For this review, take the finished solid that the model builds, in its own axes (mm). A direction names the side the tool comes from. Give positions to 0.01 mm unless a question says otherwise; leave off trailing zeros. Loops run counter-clockwise (first coordinate to the right, second up) from the corner with the lowest first, then second, coordinate; pieces in that order, holes last. Notation, with made-up numbers: (-17, 32.5) - (38, 32.5) arc R20 cw to (38, 49.5) - close; hole circle Ø4 at (-18.75, 78). An arc over 180 degrees is marked (long way). Answer as CSV lines item,"result".
Autodesk Inventor part; units mm, degrees
ref_plane "YZ Plane" through (0, 0, 0) normal (1, 0, 0) x (0, 1, 0)
ref_plane "XZ Plane" through (0, 0, 0) normal (0, 1, 0) x (-1, 0, 0)
ref_plane "XY Plane" through (0, 0, 0) normal (0, 0, 1) x (1, 0, 0)
sketch "Sketch1" plane through (0, 0, 0) normal (0, 0, 1) x (1, 0, 0)
  line L0 (0, 0) -> (18, 0)
  line L1 (18, 0) -> (18, 13)
  line L2 (18, 13) -> (12, 13)
  line L3 (12, 13) -> (12, 3)
  line L4 (12, 3) -> (0, 3)
  line L5 (0, 3) -> (0, 0) construction
  line L6 (0, 0) -> (-18, 0)
  line L7 (-18, 0) -> (-18, 13)
  line L8 (-18, 13) -> (-12, 13)
  line L9 (-12, 13) -> (-12, 3)
  line L10 (-12, 3) -> (0, 3)
  point P0 (15, 13)
  dimension "d2" = 6
  dimension "d3" = 3
  dimension "d4" = 13
  dimension "d18" = 15
extrude "Extrusion1" add sketch "Sketch1" along normal blind 12
sketch "Sketch2" plane through (-18, 0, 0) normal (0, -1, 0) x (1, 0, 0)
  circle A0 centre (18, 6) radius 1.1
  line L0 (0, 0) -> (36, 0)
  line L1 (0, 0) -> (0, 12)
  point P0 (18, 0)
  dimension "d7" = 2.2
  dimension "d19" = 6
  dimension "d20" = 18
extrude "Extrusion2" cut sketch "Sketch2" against normal blind 12
sketch "Sketch3" plane through (-12, 3, 0) normal (0, 1, 0) x (1, 0, 0)
  circle A0 centre (12, -6) radius 1.1
  circle A1 centre (12, -6) radius 4
  point P0 (12, 0)
  dimension "d11" = 8
extrude "Extrusion3" add sketch "Sketch3" along normal blind 7
sketch "Sketch5" plane through (0, 0, 0) normal (0, 0, -1) x (-1, 0, 0)
  circle A0 centre (0, 6.6873) radius 1.1
  line L0 (-12, 3) -> (12, 3)
  point P0 (0, 3)
  dimension "d29" = 2.2
extrude "Extrusion5" cut sketch "Sketch5" against normal blind 5.75
equation "\"d19\" = 0.5 * d5"
equation "\"d20\" = d18 + 0.5 * d2"
properties part number "Support_Holder" material "ABS Plastic"
1) Machinability: for faces 4 (the cylindrical face through (-1.05, 7.02, 3.43)), 5 (the cylindrical face through (2.15, 6.451, 9.373)), 6 (the flat face through (12, 8, 6)), 7 (the flat face through (15, 13, 6)), 8 (the flat face through (18, 6, 6)), which of the approach directions +Z, -Z, +X, -X, +Y, -Y give a long, thin tool a straight path to every point of the face, cutting with its end or side? Answer none if there is none.
From the geometry:
face 4,"-Z"
face 5,"+Y"
face 6,"+Z, -Z, +Y"
face 7,"+Z, -Z, +X, -X, +Y"
face 8,"+Z, -Z, +X, +Y, -Y"
2) Consider section A-A on y = 3.5. Write out the cut boundary in (x, z).
From the geometry:
outline,"(-18, 0) - (-12, 0) - (-12, 12) - (-18, 12) - close; circle Ø8 at (0, 6); (12, 0) - (18, 0) - (18, 12) - (12, 12) - close; hole circle Ø2.2 at (0, 6)"
3) Wall thickness on line 1 (X direction, y = 7, z = 6); line 2 (X direction, y = 12, z = 0.75); line 3 (X direction, y = 9.5, z = 3.75): over which ranges is each line inside the solid? List them lowest first. Write a range as from..to.
From the geometry:
line 1,"x = -18..-12, -4..-1.1, 1.1..4, 12..18"
line 2,"x = -18..-12, 12..18"
line 3,"x = -18..-12, -3.31..3.31, 12..18"
4) Draft analysis for pull direction X (two halves, no side actions). For faces 1 (the flat face through (-4, 2, 12)), 2 (the flat face through (-18, 6, 6)), 3 (the flat face through (-12, 8, 6)), state which applies: pulls with the +X half, pulls with the -X half, needs draft (parallel to the pull), parting line crosses it, or undercut.
From the geometry:
face 1,"needs draft"
face 2,"pulls with the -X half"
face 3,"undercut"
5) Consider section D-D on z = 7.5. Write out the cut boundary in (x, y), and give its area (3 significant figures).
From the geometry:
outline,"(-18, 0) - (18, 0) - (18, 13) - (12, 13) - (12, 3) - (3.71, 3) - (3.71, 10) - (-3.71, 10) - (-3.71, 3) - (-12, 3) - (-12, 13) - (-18, 13) - close"
area,"280 mm^2"
6) Insertion check: P1, Ø3, axis at x = 8, z = 4, coming from the +Y side; P2, Ø1.5, axis at x = 10.5, y = 5.5, coming from the +Z side; P3, Ø3, axis at x = 0, z = 6, coming from the +Y side; P4, Ø3, axis at x = 0, y = 6.69, coming from the +Z side. Each pin has a flat end and moves straight along its axis. Give the tip position at first contact, or say it passes through.
From the geometry:
P1,"stops at y = 3"
P2,"passes through"
P3,"stops at y = 10"
P4,"stops at z = 10"
7) Consider section B-B on x = 0. Write out the cut boundary in (y, z), and give its area (3 significant figures).
From the geometry:
outline,"(0, 0) - (3, 0) - (3, 2) - (5.59, 2) - (5.59, 4.9) - (0, 4.9) - close; (0, 7.1) - (10, 7.1) - (10, 10) - (3, 10) - (3, 12) - (0, 12) - close; (7.79, 2) - (10, 2) - (10, 4.9) - (7.79, 4.9) - close"
area,"63.6 mm^2"
8) Consider section C-C on z = 2.75. Write out the cut boundary in (x, y), and give its area (3 significant figures).
From the geometry:
outline,"(-18, 0) - (18, 0) - (18, 13) - (12, 13) - (12, 3) - (2.33, 3) - (2.33, 10) - (-2.33, 10) - (-2.33, 3) - (-12, 3) - (-12, 13) - (-18, 13) - close; hole circle Ø2.2 at (0, 6.69)"
area,"257 mm^2"
